from build123d import *

# Parameters (mm, degrees)
AUFSATZ_LINEAR_AUSTRAGEN1_DEPTH     = 75
SCHNITT_LINEAR_START                = -30
SCHNITT_LINEAR_AUSTRAGEN5_OUTLINE_W = 22.5
SCHNITT_LINEAR_AUSTRAGEN5_OUTLINE_H = 130
SCHNITT_LINEAR_AUSTRAGEN5_DEPTH     = 30


# Read off the part's stored shape, not the designer's step: Schnitt-Linear austragen5
with BuildPart() as part:
    # Skizze1 → Aufsatz-Linear austragen1 (new, symmetric)
    with BuildSketch(Plane(origin=(0, 0, 0), x_dir=(0, 0, -1), z_dir=(1, 0, 0))):
        with BuildLine():
            Line((-80, -15), (80, -15))
            ThreePointArc((80, -15), (95, 0), (80, 15))
            Line((80, 15), (-80, 15))
            ThreePointArc((-80, 15), (-95, 0), (-80, -15))
        make_face()
    extrude(amount=AUFSATZ_LINEAR_AUSTRAGEN1_DEPTH, both=True)

    # Schnitt-Linear austragen5 outline → Schnitt-Linear austragen5 (cut)
    with BuildSketch(Plane(origin=(0, 15, 0), x_dir=(1, 0, 0), z_dir=(0, 1, 0)).offset(SCHNITT_LINEAR_START)):
        with Locations((-63.75, 0)):
            Rectangle(SCHNITT_LINEAR_AUSTRAGEN5_OUTLINE_W, SCHNITT_LINEAR_AUSTRAGEN5_OUTLINE_H)
        with Locations((63.75, 0)):
            Rectangle(SCHNITT_LINEAR_AUSTRAGEN5_OUTLINE_W, SCHNITT_LINEAR_AUSTRAGEN5_OUTLINE_H)
    extrude(amount=SCHNITT_LINEAR_AUSTRAGEN5_DEPTH, mode=Mode.SUBTRACT)


solid = part.part
Work out the finished part from the listing and answer in its coordinate system (mm). A direction names the side the tool comes from. Round coordinates to 2 decimals unless told otherwise and drop trailing zeros. Write each loop counter-clockwise with the first axis right and the second up, starting at its lowest first coordinate (ties: lowest second). Pieces come first, ordered by that corner, then holes.
1) Straight lines are drawn through the part: line 1 (Z direction, x = -58, y = -1); line 2 (X direction, y = -12.5, z = 18.5); line 3 (Z direction, x = -63, y = 4.5). For each, find the intervals that lie inside material, in ascending order.
2) A cutting plane is placed at C-C (z = -60.5). Give the vertices of the cut face in (x, y), plus the area to 3 significant figures.
3) A tool of negligible diameter and unlimited length cuts with its end or side. For faces 5 (the flat face through (64, 0, -65)), 6 (the flat face through (-64, 0, 65)), 7 (the flat face through (75, 0, -80)), from which of +Z, -Z, +X, -X, +Y, -Y can it reach the whole face along a straight path? Write none if from no direction.
4) Given pin 1 Ø4 at (x, y) = (-56, 2.5) entering from -Z; pin 2 Ø2 at (y, z) = (-5, -23) entering from -X; pin 3 Ø15 at (y, z) = (6, 6) entering from +X, each flat-ended and moving along its own axis, determine where each tip first touches the part or whether it passes through.
5) A cutting plane is placed at A-A (y = 12). Give the vertices of the cut face in (x, z), plus the area to 4 significant figures.
6) The mould has two halves that part along Z. Classify faces 1 (the cylindrical face through (1, 0, 95)), 2 (the flat face through (-64, 0, -65)), 3 (the flat face through (1, -15, 1)), 4 (the flat face through (64, 0, 65)): pulls with the +Z half, pulls with the -Z half, needs draft (parallel to the pull), parting line crosses it, or undercut.
7) A cutting plane is placed at B-B (x = 7). Give the vertices of the cut face in (y, z).
8) A cutting plane is placed at D-D (y = 0). Give the vertices of the cut face in (x, z), plus the area to 4 significant figures.
Completed:
1. line 1: z = -94.97 to -65, 65 to 94.97
1. line 2: x = -52.5 to 52.5
1. line 3: z = -94.31 to -65, 65 to 94.31
2. outline: (-52.5, -15) - (52.5, -15) - (52.5, 15) - (-52.5, 15) - close
2. area: 3,150 mm2
3. face 5: +X, +Y, -Y
3. face 6: -X, +Y, -Y
3. face 7: +Z, -Z, +X, +Y, -Y
4. pin 1: stops at z = -94.99
4. pin 2: stops at x = -52.5
4. pin 3: stops at x = 52.5
5. outline: (-75, -89) - (75, -89) - (75, -65) - (52.5, -65) - (52.5, 65) - (75, 65) - (75, 89) - (-75, 89) - (-75, 65) - (-52.5, 65) - (-52.5, -65) - (-75, -65) - close
5. area: 20,850 mm2
6. face 1: pulls with the +Z half
6. face 2: undercut
6. face 3: needs draft
6. face 4: undercut
7. outline: (-15, -80) arc R15 ccw to (15, -80) - (15, 80) arc R15 ccw to (-15, 80) - close
8. outline: (-75, -95) - (75, -95) - (75, -65) - (52.5, -65) - (52.5, 65) - (75, 65) - (75, 95) - (-75, 95) - (-75, 65) - (-52.5, 65) - (-52.5, -65) - (-75, -65) - close
8. area: 22,650 mm2
